Geometry check sheet. Reference: the model listing, model coordinates, mm. Round coordinates to 2 decimals unless told otherwise and drop trailing zeros. Write each loop counter-clockwise with the first axis right and the second up, starting at its lowest first coordinate (ties: lowest second). Pieces come first, ordered by that corner, then holes. Notation, with made-up numbers: (77.25, -26.75) - (129.25, -26.75) arc R33 cw to (129.25, 11.25) - close; hole circle Ø6 at (-6.75, 53). An arc over 180 degrees is marked (long way). Return JSON: item names as keys, results as strings.
```python
from build123d import *

# Parameters (mm, degrees)
F0_W     = 42
F0_H     = 35
F1_DEPTH = 5
F2_R     = 4.99999
F3_R     = 1.5
F4_DEPTH = 6
F5_F1_R  = 1
F5_F2_R  = 1


# Not quite as in the source:
# - a fillet or chamfer is up to 0.001 mm smaller than in the source, because OpenCascade refuses the exact size


with BuildPart() as f1:
    # F0 (on Top) → F1 (new body)
    with BuildSketch(Plane.XY):
        Rectangle(F0_W, F0_H)
    extrude(amount=F1_DEPTH)

    # F2 (radius 5 in the source; OpenCascade refuses exactly that, so slightly less here)
    f2_edges = [f1.edges().sort_by_distance(p)[0] for p in [
        (-21, -17.5, 2.5),
        (21, -17.5, 2.5),
        (-21, 17.5, 2.5),
        (21, 17.5, 2.5),
        (0, 17.5, 5),
        (0, -17.5, 5),
    ]]
    fillet(f2_edges, radius=F2_R)

    # F3 (on face) → F4 (cut)
    with BuildSketch(Plane.XY.offset(5)):
        with Locations((-18, 0)):
            Circle(F3_R)
        with Locations((18, 0)):
            Circle(F3_R)
    extrude(amount=-F4_DEPTH, mode=Mode.SUBTRACT)

    # F5: fillet of radius 1 on 2 edges, made by hand

    # F5_f1
    f5_f1_edges = [f1.edges().sort_by_distance(p)[0] for p in [
        (19.5355368349, 16.0355368349, 3.5355368349),
        (21, 0, 5),
        (19.5355368349, -16.0355368349, 3.5355368349),
    ]]
    fillet(f5_f1_edges, radius=F5_F1_R)

    # F5_f2
    f5_f2_edges = [f1.edges().sort_by_distance(p)[0] for p in [
        (-19.5355368349, 16.0355368349, 3.5355368349),
        (-21, 0, 5),
        (-19.5355368349, -16.0355368349, 3.5355368349),
    ]]
    fillet(f5_f2_edges, radius=F5_F2_R)


solid = f1.part
```
(1) Section check A-A, the plane y = 0. Enter the section's corners in (x, z), plus the area to 3 significant figures.
Response values:
{"outline": "(-21, 0) - (-19.5, 0) - (-19.5, 5) - (-20, 5) arc R1 ccw to (-21, 4) - close; (-16.5, 0) - (16.5, 0) - (16.5, 5) - (-16.5, 5) - close; (19.5, 0) - (21, 0) - (21, 4) arc R1 ccw to (20, 5) - (19.5, 5) - close", "area": "180 mm^2"}
(2) Material ranges on line 1 along Y through (x, z) = (-18, 3); line 2 along X through (y, z) = (-0.5, 1.55); line 3 along X through (y, z) = (-1, 3.25), recorded low to high. Write a range as [from, to].
Response values:
{"line 1": "y = [-16.5, -1.5], [1.5, 16.5]", "line 2": "x = [-21, -19.41], [-16.59, 16.59], [19.41, 21]", "line 3": "x = [-21, -19.12], [-16.88, 16.88], [19.12, 21]"}
(3) Section check C-C, the plane z = 1.5. Give the number of separate pieces and of enclosed holes in the cut face, plus the area to 3 significant figures.
Response values:
{"separate pieces": "1", "enclosed holes": "2", "area": "1,420 mm^2"}
(4) Gauge pin test, flat end, axial feed: pin 1 (2 mm diameter, centred on y = -14, z = 1.5, fed in from +X). Record the tip position at first contact, or that the pin passes through.
Response values:
{"pin 1": "stops at x = 20.97"}
(5) Release check for a two-part mould opening along X. For faces 1 (the face through (0, 0, 0)), 2 (the face through (16.5, 0.07, 2.54)), 3 (the face through (20.13, 15.32, 1.58)) record: pulls with the +X half, pulls with the -X half, needs draft (parallel to the pull), parting line crosses it, or undercut.
Response values:
{"face 1": "needs draft", "face 2": "undercut", "face 3": "pulls with the +X half"}
